Read the model definition and answer for the solid it produces. Units are mm, in the model's axes. A direction names the side the tool comes from. Give positions to 0.01 mm unless a question says otherwise; leave off trailing zeros. Loops run counter-clockwise (first coordinate to the right, second up) from the corner with the lowest first, then second, coordinate; pieces in that order, holes last. Notation, with made-up numbers: (-6.5, -6) - (7.5, -6) arc R29 ccw to (7.5, 19) - close; hole circle Ø2 at (-38, 14.5). An arc over 180 degrees is marked (long way). Use a Markdown table: item, result. Add a question column.
Item 1: A cutting plane is placed at D-D (x = 10.5). Determine the outline of the cut face in (y, z), plus the area to 3 significant figures.
Item 2: For a pull along Z with two mould halves and no side action, classify faces 4 (the face through (0, -45, 0)), 5 (the face through (-20, -15, 29)), 6 (the face through (0, -20, -33.5)) as +Z half, -Z half, draft (parallel to the pull), parting line (faces both ways), or undercut.
Item 3: A cutting plane is placed at C-C (y = -34.5). Determine the outline of the cut face in (x, z), plus the area to 3 significant figures.
Item 4: Consider probe 1 along Z at (x, y) = (-18, -14); probe 2 along X at (y, z) = (0, -29.5); probe 3 along Y at (x, z) = (0, 26.5). Determine where each line is inside the solid, lowest interval first. Write a range as [from, to].
Item 5: Each of these flat-tipped pins is pushed along its axis until it touches: P1, Ø4.5, axis at y = -6, z = -30, coming from the -X side; P2, Ø10, axis at y = -21.5, z = -29, coming from the +X side; P3, Ø6, axis at x = -8.5, z = -9.5, coming from the +Y side. Where does it stop, or does it pass through?
Item 6: Which of the six approach directions +Z, -Z, +X, -X, +Y, -Y give full straight-line access (tool end or side, diameter ignored) to faces 1 (the face through (20, -15, -29)), 2 (the face through (0, -15, -24.5)), 3 (the face through (-20, -15, -29))?
Item 7: A cutting plane is placed at B-B (y = 0). Determine the outline of the cut face in (x, z).
Item 8: A cutting plane is placed at A-A (x = 0). Determine the outline of the cut face in (y, z), plus the area to 3 significant figures.
from build123d import *

# Parameters (mm, degrees)
SKETCH2_W               = 70
SKETCH2_H               = 10
BOSS_EXTRUDE1_DEPTH     = 33.5
SKETCH3_W               = 40
SKETCH3_H               = 60
BOSS_EXTRUDE2_DEPTH     = 33.5
SKETCH4_W               = 40
SKETCH4_H               = 60
CUT_EXTRUDE1_DEPTH      = 24.5
CUT_EXTRUDE2_DEPTH      = 74.295634249
CUT_EXTRUDE2_DEPTH_BACK = 74.295634249
SKETCH5_R               = 7.6


with BuildPart() as part:
    # Sketch2 → Boss-Extrude1 (new, symmetric)
    with BuildSketch(Plane.XY):
        with Locations((0, -50)):
            Rectangle(SKETCH2_W, SKETCH2_H)
    extrude(amount=BOSS_EXTRUDE1_DEPTH, both=True)

    # Sketch3 → Boss-Extrude2 (add, symmetric)
    with BuildSketch(Plane.XY):
        with Locations((0, -15)):
            Rectangle(SKETCH3_W, SKETCH3_H)
    extrude(amount=BOSS_EXTRUDE2_DEPTH, both=True)

    # Sketch4 → Cut-Extrude1 (cut, symmetric)
    with BuildSketch(Plane.XY):
        with Locations((0, -15)):
            Rectangle(SKETCH4_W, SKETCH4_H)
    extrude(amount=CUT_EXTRUDE1_DEPTH, both=True, mode=Mode.SUBTRACT)

    # Sketch5 → Cut-Extrude2 (cut, two sides: drawn at the far end of the back side and taken through both)
    with BuildSketch(Plane.XY.offset(-CUT_EXTRUDE2_DEPTH_BACK)):
        Circle(SKETCH5_R)
    extrude(amount=CUT_EXTRUDE2_DEPTH + CUT_EXTRUDE2_DEPTH_BACK, mode=Mode.SUBTRACT)


solid = part.part
Geometry says:
| question | item | result |
|---|---|---|
| 1 | outline | (-55, -33.5) - (15, -33.5) - (15, -24.5) - (-45, -24.5) - (-45, 24.5) - (15, 24.5) - (15, 33.5) - (-55, 33.5) - close |
| 1 | area | 1,750 mm² |
| 2 | face 4 | undercut |
| 2 | face 5 | draft |
| 2 | face 6 | -Z half |
| 3 | outline | (-20, -33.5) - (20, -33.5) - (20, -24.5) - (-20, -24.5) - close; (-20, 24.5) - (20, 24.5) - (20, 33.5) - (-20, 33.5) - close |
| 3 | area | 720 mm² |
| 4 | probe 1 | [-33.5, -24.5], [24.5, 33.5] |
| 4 | probe 2 | [-20, -7.6], [7.6, 20] |
| 4 | probe 3 | [-55, -7.6], [7.6, 15] |
| 5 | P1 | x = -20 |
| 5 | P2 | x = 20 |
| 5 | P3 | y = -45 |
| 6 | face 1 | +Z, -Z, +X, +Y |
| 6 | face 2 | +X, -X, +Y |
| 6 | face 3 | +Z, -Z, -X, +Y |
| 7 | outline | (-20, -33.5) - (-7.6, -33.5) - (-7.6, -24.5) - (-20, -24.5) - close; (-20, 24.5) - (-7.6, 24.5) - (-7.6, 33.5) - (-20, 33.5) - close; (7.6, -33.5) - (20, -33.5) - (20, -24.5) - (7.6, -24.5) - close; (7.6, 24.5) - (20, 24.5) - (20, 33.5) - (7.6, 33.5) - close |
| 8 | outline | (-55, -33.5) - (-7.6, -33.5) - (-7.6, -24.5) - (-45, -24.5) - (-45, 24.5) - (-7.6, 24.5) - (-7.6, 33.5) - (-55, 33.5) - close; (7.6, -33.5) - (15, -33.5) - (15, -24.5) - (7.6, -24.5) - close; (7.6, 24.5) - (15, 24.5) - (15, 33.5) - (7.6, 33.5) - close |
| 8 | area | 1,480 mm² |
